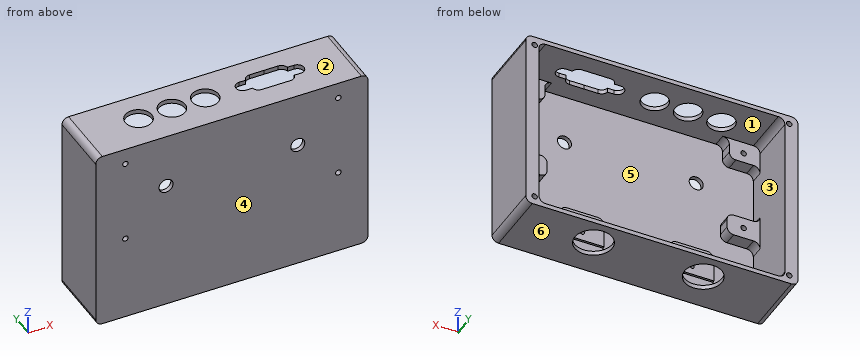
from build123d import *

# Parameters (mm, degrees)
SKIZZE1_W                       = 116
SKIZZE1_H                       = 85
AUFSATZ_LINEAR_AUSTRAGEN1_DEPTH = 30
SCHALE1_T                       = -2
SKIZZE2_R                       = 6
SCHNITT_LINEAR_AUSTRAGEN1_DEPTH = 30
SCHNITT_LINEAR_AUSTRAGEN2_DEPTH = 10
VERRUNDUNG1_R                   = 3
AUFSATZ_LINEAR_AUSTRAGEN2_DEPTH = 6
VERRUNDUNG2_R                   = 3
SKIZZE5_W                       = 15
SKIZZE5_H                       = 10
AUFSATZ_LINEAR_AUSTRAGEN3_DEPTH = 6
VERRUNDUNG3_R                   = 3
SKIZZE6_R                       = 8.5
SCHNITT_LINEAR_AUSTRAGEN3_DEPTH = 5
SKIZZE7_W                       = 20
SKIZZE7_H                       = 20
AUFSATZ_LINEAR_AUSTRAGEN4_DEPTH = 6
VERRUNDUNG4_R                   = 3
M3_GEWINDEBOHRUNG1_D            = 2.5
M3_GEWINDEBOHRUNG1_DEPTH        = 8.5
M3_GEWINDEBOHRUNG1_TIP          = 0.751075774
M2_5_GEWINDEBOHRUNG1_D          = 2.05
M2_5_GEWINDEBOHRUNG1_DEPTH      = 7.25
M2_5_GEWINDEBOHRUNG1_TIP        = 0.615882135
SKIZZE12_W                      = 90
SKIZZE12_H                      = 6
SCHNITT_LINEAR_AUSTRAGEN4_DEPTH = 1
SKIZZE13_R                      = 3.2
SCHNITT_LINEAR_AUSTRAGEN5_DEPTH = 10
AUFSATZ_LINEAR_START            = -30
AUFSATZ_LINEAR_AUSTRAGEN5_DEPTH = 30
VERRUNDUNG5_R                   = 3
M3_GEWINDEBOHRUNG2_D            = 2.5
M3_GEWINDEBOHRUNG2_DEPTH        = 8.5
M3_GEWINDEBOHRUNG2_TIP          = 0.751075774


with BuildPart() as part:
    # Skizze1 → Aufsatz-Linear austragen1 (new body)
    with BuildSketch(Plane(origin=(0, 0, 0), x_dir=(1, 0, 0), z_dir=(0, 1, 0))):
        with Locations((58, 42.5)):
            Rectangle(SKIZZE1_W, SKIZZE1_H)
    extrude(amount=AUFSATZ_LINEAR_AUSTRAGEN1_DEPTH)

    # Schale1
    schale1_openings = [part.faces().sort_by_distance(p)[0] for p in [
        (58, 30, -42.5),
    ]]
    offset(amount=SCHALE1_T, openings=schale1_openings, kind=Kind.INTERSECTION)

    # Skizze2 → Schnitt-Linear austragen1 (cut)
    with BuildSketch(Plane.XY):
        with Locations((23.64, 15.94)):
            Circle(SKIZZE2_R)
        with Locations((38.84, 15.94)):
            Circle(SKIZZE2_R)
        with Locations((54.04, 15.94)):
            Circle(SKIZZE2_R)
    extrude(amount=-SCHNITT_LINEAR_AUSTRAGEN1_DEPTH, mode=Mode.SUBTRACT)

    # Skizze3 → Schnitt-Linear austragen2 (cut)
    with BuildSketch(Plane.XY):
        with BuildLine():
            ThreePointArc((90.082181292, 21.48963825), (92.018633773, 20.780819017), (93.040082938, 18.989474685))
            Line((93.040082938, 18.989474685), (96.04016588, 18.989308791))
            ThreePointArc((96.04016588, 18.989308791), (99.039999986, 15.989142906), (96.039834101, 12.9893088))
            Line((96.039834101, 12.9893088), (93.03975116, 12.989474694))
            ThreePointArc((93.03975116, 12.989474694), (92.018103892, 11.198243337), (90.081573032, 10.489638266))
            Line((90.081573032, 10.489638266), (83.54015207, 10.49))
            Line((83.54015207, 10.49), (76.998122837, 10.49))
            ThreePointArc((76.998122837, 10.49), (75.061631164, 11.198712153), (74.040082946, 12.99))
            Line((74.040082946, 12.99), (71.04, 12.99))
            ThreePointArc((71.04, 12.99), (68.04, 15.99), (71.04, 18.99))
            Line((71.04, 18.99), (74.040082946, 18.99))
            ThreePointArc((74.040082946, 18.99), (75.061631164, 20.781287847), (76.998122837, 21.49))
            Line((76.998122837, 21.49), (83.54015207, 21.49))
            Line((83.54015207, 21.49), (90.082181292, 21.48963825))
        make_face()
    extrude(amount=-SCHNITT_LINEAR_AUSTRAGEN2_DEPTH, mode=Mode.SUBTRACT)

    # Verrundung1
    verrundung1_edges = [part.edges().sort_by_distance(p)[0] for p in [
        (2, 16, -83),
        (2, 16, -2),
        (114, 16, -2),
        (114, 16, -83),
        (0, 15, -85),
        (116, 15, -85),
        (116, 15, 0),
        (0, 15, 0),
    ]]
    fillet(verrundung1_edges, radius=VERRUNDUNG1_R)

    # Skizze4 → Aufsatz-Linear austragen2 (add)
    with BuildSketch(Plane(origin=(0, 2, 0), x_dir=(1, 0, 0), z_dir=(0, 1, 0))):
        with BuildLine():
            Line((13, 12), (2, 12))
            Line((2, 12), (2, 5))
            ThreePointArc((2, 5), (2.878679656, 2.878679656), (5, 2))
            Line((5, 2), (16, 2))
            Line((16, 2), (16, 9))
            ThreePointArc((16, 9), (15.121320344, 11.121320344), (13, 12))
        make_face()
        with BuildLine():
            Line((100, 9), (100, 2))
            Line((100, 2), (111, 2))
            ThreePointArc((111, 2), (113.121320344, 2.878679656), (114, 5))
            Line((114, 5), (114, 12))
            Line((114, 12), (103, 12))
            ThreePointArc((103, 12), (100.878679656, 11.121320344), (100, 9))
        make_face()
    extrude(amount=AUFSATZ_LINEAR_AUSTRAGEN2_DEPTH)

    # Verrundung2
    verrundung2_edges = [part.edges().sort_by_distance(p)[0] for p in [
        (2, 5, -12),
        (16, 5, -2),
        (114, 5, -12),
        (100, 5, -2),
    ]]
    fillet(verrundung2_edges, radius=VERRUNDUNG2_R)

    # Skizze5 → Aufsatz-Linear austragen3 (add)
    with BuildSketch(Plane(origin=(0, 2, 0), x_dir=(1, 0, 0), z_dir=(0, 1, 0))):
        with Locations((9.5, 45.4)):
            Rectangle(SKIZZE5_W, SKIZZE5_H)
        with Locations((106.5, 45.4)):
            Rectangle(SKIZZE5_W, SKIZZE5_H)
    extrude(amount=AUFSATZ_LINEAR_AUSTRAGEN3_DEPTH)

    # Verrundung3
    verrundung3_edges = [part.edges().sort_by_distance(p)[0] for p in [
        (2, 5, -50.4),
        (2, 5, -40.4),
        (17, 5, -40.4),
        (17, 5, -50.4),
        (114, 5, -50.4),
        (99, 5, -50.4),
        (99, 5, -40.4),
        (114, 5, -40.4),
    ]]
    fillet(verrundung3_edges, radius=VERRUNDUNG3_R)

    # Skizze6 → Schnitt-Linear austragen3 (cut)
    with BuildSketch(Plane(origin=(0, 0, -85), x_dir=(-1, 0, 0), z_dir=(0, 0, -1))):
        with Locations((-83, 18)):
            Circle(SKIZZE6_R)
        with Locations(Location((-33, 18, 0), (0, 0, 180))):
            Circle(SKIZZE6_R)
    extrude(amount=-SCHNITT_LINEAR_AUSTRAGEN3_DEPTH, mode=Mode.SUBTRACT)

    # Skizze7 → Aufsatz-Linear austragen4 (add)
    with BuildSketch(Plane(origin=(0, 2, 0), x_dir=(1, 0, 0), z_dir=(0, 1, 0))):
        with Locations((33, 73)):
            Rectangle(SKIZZE7_W, SKIZZE7_H)
        with Locations((83, 73)):
            Rectangle(SKIZZE7_W, SKIZZE7_H)
    extrude(amount=AUFSATZ_LINEAR_AUSTRAGEN4_DEPTH)

    # Verrundung4
    verrundung4_edges = [part.edges().sort_by_distance(p)[0] for p in [
        (23, 5, -63),
        (43, 5, -63),
        (43, 5, -83),
        (23, 5, -83),
        (73, 5, -63),
        (93, 5, -63),
        (93, 5, -83),
        (73, 5, -83),
    ]]
    fillet(verrundung4_edges, radius=VERRUNDUNG4_R)

    # M3 Gewindebohrung1
    with Locations(Plane(origin=(0, 8, 0), x_dir=(1, 0, 0), z_dir=(0, 1, 0))):
        with Locations((106.5, 7.4), (9.5, 45.4), (106.5, 45.4), (9.5, 7.4)):
            Hole(M3_GEWINDEBOHRUNG1_D / 2, depth=M3_GEWINDEBOHRUNG1_DEPTH)
            with Locations((0, 0, -(M3_GEWINDEBOHRUNG1_DEPTH + M3_GEWINDEBOHRUNG1_TIP / 2))):  # 118° drill point
                Cone(0, M3_GEWINDEBOHRUNG1_D / 2, M3_GEWINDEBOHRUNG1_TIP, mode=Mode.SUBTRACT)

    # M2.5 Gewindebohrung1
    with Locations(Plane(origin=(0, 8, 0), x_dir=(1, 0, 0), z_dir=(0, 1, 0))):
        with Locations((33, 73), (83, 73)):
            Hole(M2_5_GEWINDEBOHRUNG1_D / 2, depth=M2_5_GEWINDEBOHRUNG1_DEPTH)
            with Locations((0, 0, -(M2_5_GEWINDEBOHRUNG1_DEPTH + M2_5_GEWINDEBOHRUNG1_TIP / 2))):  # 118° drill point
                Cone(0, M2_5_GEWINDEBOHRUNG1_D / 2, M2_5_GEWINDEBOHRUNG1_TIP, mode=Mode.SUBTRACT)

    # Skizze12 → Schnitt-Linear austragen4 (cut)
    with BuildSketch(Plane(origin=(0, 8, 0), x_dir=(1, 0, 0), z_dir=(0, 1, 0))):
        with Locations((63.848936769, 80)):
            Rectangle(SKIZZE12_W, SKIZZE12_H)
    extrude(amount=-SCHNITT_LINEAR_AUSTRAGEN4_DEPTH, mode=Mode.SUBTRACT)

    # Skizze13 → Schnitt-Linear austragen5 (cut)
    with BuildSketch(Plane(origin=(0, 2, 0), x_dir=(1, 0, 0), z_dir=(0, 1, 0))):
        with Locations(Location((88, 25, 0), (0, 0, 270))):
            Circle(SKIZZE13_R)
        with Locations(Location((28, 25, 0), (0, 0, 90))):
            Circle(SKIZZE13_R)
    extrude(amount=-SCHNITT_LINEAR_AUSTRAGEN5_DEPTH, mode=Mode.SUBTRACT)

    # Skizze14 → Aufsatz-Linear austragen5 (add)
    with BuildSketch(Plane(origin=(0, 0, 0), x_dir=(-1, 0, 0), z_dir=(0, -1, 0)).offset(AUFSATZ_LINEAR_START)):
        with BuildLine():
            Line((-116, 0), (-120, 0))
            Line((-120, 0), (-120, 85))
            Line((-120, 85), (-116, 85))
            Line((-116, 85), (-113, 85))
            ThreePointArc((-113, 85), (-115.121320344, 84.121320344), (-116, 82))
            Line((-116, 82), (-116, 3))
            ThreePointArc((-116, 3), (-115.121320344, 0.878679656), (-113, 0))
            Line((-113, 0), (-116, 0))
        make_face()
        with BuildLine():
            Line((0, 85), (4, 85))
            Line((4, 85), (4, 0))
            Line((4, 0), (0, 0))
            Line((0, 0), (-3, 0))
            ThreePointArc((-3, 0), (-0.878679656, 0.878679656), (0, 3))
            Line((0, 3), (0, 82))
            ThreePointArc((0, 82), (-0.878679656, 84.121320344), (-3, 85))
            Line((-3, 85), (0, 85))
        make_face()
    extrude(amount=AUFSATZ_LINEAR_AUSTRAGEN5_DEPTH)

    # Verrundung5
    verrundung5_edges = [part.edges().sort_by_distance(p)[0] for p in [
        (120, 15, 0),
        (120, 15, -85),
        (-4, 15, -85),
        (-4, 15, 0),
    ]]
    fillet(verrundung5_edges, radius=VERRUNDUNG5_R)

    # M3 Gewindebohrung2
    with Locations(Plane(origin=(0, 30, 0), x_dir=(1, 0, 0), z_dir=(0, 1, 0))):
        with Locations((0, 4), (116, 81), (0, 81), (116, 4)):
            Hole(M3_GEWINDEBOHRUNG2_D / 2, depth=M3_GEWINDEBOHRUNG2_DEPTH)
            with Locations((0, 0, -(M3_GEWINDEBOHRUNG2_DEPTH + M3_GEWINDEBOHRUNG2_TIP / 2))):  # 118° drill point
                Cone(0, M3_GEWINDEBOHRUNG2_D / 2, M3_GEWINDEBOHRUNG2_TIP, mode=Mode.SUBTRACT)


solid = part.part
Verification items for the finished model (mm, model axes). Face numbers are marked on the shaded views. A direction names the side the tool comes from. Round coordinates to 2 decimals unless told otherwise and drop trailing zeros. Order: outer loops, then holes, each group sorted by start corner. A loop starts at its lowest first (then second) coordinate and runs counter-clockwise, first axis right, second up. Notation, with made-up numbers: (84.25, 23) -> (102.25, 23) arc R31 cw to (102.25, 47) -> close; hole circle Ø6 at (26.25, 36). An arc over 180 degrees is marked (long way). Put each result on its own line as item: value.
1) Mould release check, pull along Z, two halves, no side actions. Record for the marked faces 1, 2, 3 and 4: +Z half, -Z half, draft (parallel to the pull), parting line (faces both ways), or undercut.
Final values:
face 1: undercut
face 2: +Z half
face 3: undercut
face 4: draft
2) Section check C-C (x = 28). Record the cut outline in (y, z).
Final values:
outline: (0, -85) -> (11.13, -85) -> (11.13, -83) -> (7, -83) -> (7, -77) -> (8, -77) -> (8, -63) -> (2, -63) -> (2, -28.2) -> (0, -28.2) -> close; (0, -21.8) -> (2, -21.8) -> (2, -2) -> (11.82, -2) -> (11.82, 0) -> (0, 0) -> close; (20.06, -2) -> (30, -2) -> (30, 0) -> (20.06, 0) -> close; (24.87, -85) -> (30, -85) -> (30, -83) -> (24.87, -83) -> close
3) Material ranges on line 1 (Z direction, x = 0, y = 24.25); line 2 (X direction, y = 6.25, z = -7.4); line 3 (X direction, y = 6.75, z = -73) (3 decimals), recorded low to high.
Final values:
line 1: z = -85 to -82.25, -79.75 to -5.25, -2.75 to 0
line 2: x = -4 to 8.25, 10.75 to 16, 100 to 105.25, 107.75 to 120
line 3: x = -4 to 2, 23 to 31.975, 34.025 to 43, 73 to 81.975, 84.025 to 93, 114 to 120
4) Section check D-D (y = 4.75). Give the number of separate pieces and of enclosed holes in the cut face, then the cut area to 3 significant figures.
Final values:
separate pieces: 1
enclosed holes: 7
area: 2,820 mm^2
5) Section check B-B (z = -56). Record the cut outline in (x, y).
Final values:
outline: (-4, 0) -> (120, 0) -> (120, 30) -> (114, 30) -> (114, 2) -> (2, 2) -> (2, 30) -> (-4, 30) -> close
6) Depth check by flat-ended pin: pin 1 (3 mm diameter, centred on x = 84.5, y = 13.5, fed in from +Z); pin 2 (3 mm diameter, centred on x = 106.5, z = -45.4, fed in from +Y); pin 3 (11 mm diameter, centred on x = 38.84, y = 15.94, fed in from +Z). Enter the tip coordinate at first touch or a pass-through.
Final values:
pin 1: passes through
pin 2: stops at y = 8
pin 3: stops at z = -83
7) Section check A-A (x = 106.5). Record the cut outline in (y, z).
Final values:
outline: (0, -85) -> (30, -85) -> (30, -83) -> (2, -83) -> (2, -50.4) -> (8, -50.4) -> (8, -46.65) -> (0, -46.65) -> close; (0, -44.15) -> (8, -44.15) -> (8, -40.4) -> (2, -40.4) -> (2, -12) -> (8, -12) -> (8, -8.65) -> (0, -8.65) -> close; (0, -6.15) -> (8, -6.15) -> (8, -2) -> (30, -2) -> (30, 0) -> (0, 0) -> close
8) Set-up check for the marked faces 5 and 6: record each of +Z, -Z, +X, -X, +Y, -Y from which the full face is reachable in a straight line by a thin tool's end or side.
Final values:
face 5: +Y
face 6: -Z, +X, -X, +Y, -Y
